Autodesk Inventor part; units mm, degrees
ref_plane "YZ Plane" through (0, 0, 0) normal (1, 0, 0) x (0, 1, 0)
ref_plane "XZ Plane" through (0, 0, 0) normal (0, 1, 0) x (-1, 0, 0)
ref_plane "XY Plane" through (0, 0, 0) normal (0, 0, 1) x (1, 0, 0)
sketch "スケッチ1" plane through (0, 0, 0) normal (0, 0, 1) x (1, 0, 0)
  circle A0 centre (-73.413, 50.8387) radius 2
  circle A1 centre (-11.7367, 127.3646) radius 2
  circle A2 centre (-32.2967, 116.5802) radius 2
  circle A3 centre (-53.1365, 95) radius 5.025
  circle A4 centre (-11.7367, 127.3646) radius 6
  circle A5 centre (-32.2967, 116.5802) radius 6
  circle A6 centre (-53.1365, 95) radius 11.5
  circle A7 centre (-73.413, 50.8387) radius 6
  line L0 (-79.114, 52.7091) -> (-64.0635, 98.5848)
  line L1 (-59.8041, 104.3698) -> (-35.7755, 121.4688)
  line L2 (-35.0838, 121.8936) -> (-14.5238, 132.678)
  line L3 (-29.5097, 111.2668) -> (-8.9496, 122.0512)
  line L4 (-27.2897, 113.2742) -> (-43.5397, 88.6634)
  line L5 (-43.2957, 89.0494) -> (-68.2786, 47.734)
  circle A8 centre (-53.1365, 95) radius 7.5
  point P0 (0, 0)
  point P1 (-43.4139, 88.854)
  point P2 (-28.1412, 111.9846)
  dimension "d0" = 4
  dimension "d1" = 4
  dimension "d2" = 4
  dimension "d3" = 10.05
  dimension "d4" = 4
  dimension "d5" = 4
  dimension "d7" = 4
  dimension "d15" = 15
  dimension "d16" = 4
extrude "押し出し1" add sketch "スケッチ1" along normal blind 3 contours A4 | A4 L3 L4 A5 L2 | A5 | L4 L5 A6 L1 A5 L3 | L3 A5 L4 | L5 A7 L0 A6 L4 | L4 A6 L5 | A6 | A7 | A8
sketch "スケッチ2" plane through (0, 0, 0) normal (0, 0, -1) x (-1, 0, 0)
  circle A0 centre (53.1365, 95) radius 5.025
  circle A1 centre (53.1365, 95) radius 7.5
  point P0 (0, 0)
  dimension "d12" = 15
extrude "押し出し2" cut sketch "スケッチ2" against normal blind 0.5
shell "シェル2" thickness 3 removed faces 2 at (-67.6516, 80.9362, 0) at (-66.6917, 80.9872, 3)
fillet "フィレット2" radius 1 19 edges at (-43.4139, 88.854, 1.5) (-28.1412, 111.9846, 1.5) (-75.0166, 55.5746, 1.5) (-63.1345, 91.7924, 1.75) (-63.1345, 91.7924, 0.25) (-68.776, 52.7092, 1.5) (-49.0526, 85.3267, 0.25) (-49.0526, 85.3267, 1.75) (-45.6365, 95, 0.5) (-53.0422, 105.4996, 0.25) (-53.0422, 105.4996, 1.75) (-37.2952, 116.7053, 1.5) (-42.6466, 95.4607, 0.25) (-31.9972, 111.5892, 1.5) (-42.6466, 95.4607, 1.75) (-30.148, 121.0949, 1.5) (-16.6725, 128.1633, 1.5) (-27.3609, 115.7815, 1.5) (-13.8854, 122.8499, 1.5)
sketch "スケッチ3" plane through (0, 0, 0) normal (0, 0, -1) x (-1, 0, 0)
  circle A0 centre (53.1365, 95) radius 5.025
  circle A1 centre (53.1365, 95) radius 7.5
  point P0 (0, 0)
  dimension "d19" = 15
extrude "押し出し3" cut sketch "スケッチ3" against normal blind 0.5 contours A0 | A1
properties part number "アーム軸抑え3" material "アルミニウム 2014-T4"
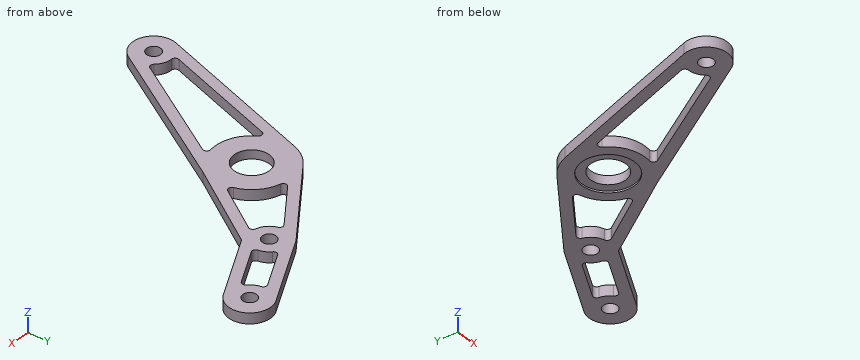
The listing builds one solid part. Answer for the finished solid, in the listing's coordinates (mm). Round coordinates to 2 decimals unless told otherwise and drop trailing zeros. Loops run counter-clockwise (first coordinate to the right, second up) from the corner with the lowest first, then second, coordinate; pieces in that order, holes last. Notation, with made-up numbers: M 79.25,-3.5 L 86.25,-3.5 A24 ccw 86.25,33.5 Z; hole C -39.75,79 d3. An arc over 180 degrees is marked long. Return JSON: item names as keys, results as strings.
Q1. Each of these flat-tipped pins is pushed along its axis until it touches: pin 1 Ø1 at (x, z) = (-40.5, 2.5) entering from -Y; pin 2 Ø13.5 at (x, y) = (-53.14, 95) entering from -Z. Where does it stop, or does it pass through?
Results list:
{"pin 1": "stops at y = 92.51", "pin 2": "stops at z = 0.5"}
Q2. Find section D-D, the plane z = 1.65. State how many separate pieces and enclosed holes the cut face has, plus the area to 3 significant figures.
Results list:
{"separate pieces": "1", "enclosed holes": "7", "area": "1,040 mm2"}
Q3. Find the intervals of material crossed by line 1 along Y through (x, z) = (-49, 0.3); line 2 along X through (y, z) = (126, 0.7); line 3 along X through (y, z) = (122, 1.8), in increasing order. Write a range as from..to.
Results list:
{"line 1": "y = 79.62..88.74, 101.26..104.65, 108.38..112.06", "line 2": "x = -27.26..-20.8, -16.55..-13.2, -10.27..-5.89", "line 3": "x = -34.88..-28.42, -15.51..-9.05"}
Q4. Find section A-A, the plane y = 62.5. Determine the outline of the cut face in (x, z), plus the area to 3 significant figures.
Results list:
{"outline": "M -75.9,0 L -72.74,0 L -72.74,3 L -75.9,3 Z; M -62.86,0 L -59.35,0 L -59.35,3 L -62.86,3 Z", "area": "20.0 mm2"}
Q5. Find section C-C, the plane y = 108. Determine the outline of the cut face in (x, z).
Results list:
{"outline": "M -54.7,0 L -49.53,0 L -49.53,3 L -54.7,3 Z; M -34.37,0 L -30.77,0 L -30.77,3 L -34.37,3 Z"}
Q6. Find section B-B, the plane x = -53. Determine the outline of the cut face in (y, z).
Results list:
{"outline": "M 73,0 L 78.8,0 L 78.8,3 L 73,3 Z; M 84.5,0 L 87.5,0 L 87.5,0.5 L 89.98,0.5 L 89.98,3 L 84.5,3 Z; M 100.02,0.5 L 102.5,0.5 L 102.5,0 L 109.21,0 L 109.21,3 L 100.02,3 Z"}
